Autodesk Inventor part; units mm, degrees
ref_plane "Work Plane1" through (0, 0, -15) normal (0, 0, 1) x (1, 0, 0)
ref_plane "YZ Plane" through (0, 0, 0) normal (1, 0, 0) x (0, 1, 0)
ref_plane "XZ Plane" through (0, 0, 0) normal (0, 1, 0) x (-1, 0, 0)
sketch "Sketch1" plane through (0, 0, 0) normal (0, 0, 1) x (1, 0, 0)
  line L0 (0, 0) -> (25, 0)
  line L1 (25, 0) -> (25, 40)
  line L2 (25, 40) -> (0, 40)
  line L3 (0, 40) -> (0, 0)
  dimension "d1" = 25
  dimension "d2" = 40
  dimension "d3" = 25
extrude "Extrusion1" add sketch "Sketch1" against normal blind 30
sketch "Sketch2" plane through (25, 0, 0) normal (1, 0, 0) x (0, 0, -1)
  line L0 (0, 0) -> (30, 0)
  circle A0 centre (15, 6.56) radius 2.46
extrude "Extrusion2" cut sketch "Sketch2" against normal blind 30
sketch "Sketch3" plane through (0, 0, 0) normal (-1, 0, 0) x (0, 0, 1)
  line L0 (0, 0) -> (-30, 0)
  line L1 (-25.05, 0) -> (-4.95, 0)
  line L2 (-4.95, 0) -> (-4.95, 33.12)
  line L3 (-4.95, 33.12) -> (-25.05, 33.12)
  line L4 (-25.05, 33.12) -> (-25.05, 0)
  dimension "d11" = 20.1
extrude "Extrusion3" cut sketch "Sketch3" against normal blind 20
sketch "Sketch4" plane through (0, 0, 0) normal (0, -1, 0) x (1, 0, 0)
  line L0 (20, -4.95) -> (20, -25.05)
  line L1 (20, -15) -> (25, -15)
  line L2 (25, 0) -> (25, -30)
  line L3 (20, -8.025) -> (25, -8.025)
  line L4 (25, -8.025) -> (25, -21.975)
  line L5 (25, -21.975) -> (20, -21.975)
  line L6 (20, -21.975) -> (20, -8.025)
  line L7 (20, -8.025) -> (25, -21.975) construction
  line L8 (25, -8.025) -> (20, -21.975) construction
  line L9 (25, -12.54) -> (25, -17.46)
  point P0 (0, 0)
  point P1 (22.5, -15)
  dimension "d14" = 13.95
extrude "Extrusion4" add sketch "Sketch4" along normal blind 15
sketch "Sketch5" plane through (20, 0, 0) normal (-1, 0, 0) x (0, 0, 1)
  circle A0 centre (-15, 6.56) radius 2.46
  circle A1 centre (-15, 6.56) radius 4.7025
  circle A2 centre (-15, 6.56) radius 2.46
  circle A3 centre (-15, 6.56) radius 2.46
  point P0 (0, 0)
  dimension "d17" = 9.405
extrude "Extrusion5" cut sketch "Sketch5" against normal blind 2.1
sketch "Sketch6" plane through (25, 0, 0) normal (1, 0, 0) x (0, 0, -1)
  circle A0 centre (15, 6.56) radius 4.7025
  line L0 (15, 6.56) -> (15, 23.56)
  circle A1 centre (15, 23.56) radius 2.46
  point P0 (0, 0)
  dimension "d20" = 17
  dimension "d21" = 4.92
extrude "Extrusion6" cut sketch "Sketch6" against normal blind 10 contours A1
sketch "Sketch7" plane through (20, 0, 0) normal (-1, 0, 0) x (0, 0, 1)
  circle A0 centre (-15, 23.56) radius 2.46
  circle A1 centre (-15, 23.56) radius 4.7025
  point P0 (0, 0)
  dimension "d24" = 9.405
extrude "Extrusion7" cut sketch "Sketch7" against normal blind 2.1
sketch "Sketch9" plane through (25, 0, 0) normal (1, 0, 0) x (0, 0, -1)
  circle A0 centre (15, 6.56) radius 2.46
  circle A1 centre (15, 6.56) radius 2.46
  circle A2 centre (15, 23.56) radius 2.46
  circle A3 centre (15, 23.56) radius 2.46
  line L0 (30, 40) -> (30, 0)
  line L1 (30, 0) -> (30, 40)
  line L2 (30, 40) -> (0, 40)
  line L3 (0, 40) -> (0, 0)
  line L4 (0, 0) -> (8.025, 0)
  line L5 (21.975, 0) -> (21.975, -15)
  line L6 (21.975, -15) -> (8.025, -15)
  line L7 (8.025, -15) -> (8.025, 0)
  line L8 (0, 0) -> (8.025, 0)
  line L9 (21.975, 0) -> (30, 0)
extrude "Extrusion8" add sketch "Sketch9" along normal blind 5
sketch "Sketch10" plane through (0, 40, 0) normal (0, 1, 0) x (1, 0, 0)
  line L0 (0, 30) -> (30, 30)
  line L1 (30, 0) -> (0, 0)
  line L2 (0, 30) -> (30, 30)
  line L3 (30, 30) -> (30, 0)
  line L4 (30, 0) -> (0, 0)
  line L5 (0, 0) -> (0, 30)
extrude "Extrusion9" add sketch "Sketch10" along normal blind 30
sketch "Sketch12" plane through (30, 0, 0) normal (1, 0, 0) x (0, 0, -1)
  circle A0 centre (15, 6.56) radius 2.46
  line L0 (15, 6.56) -> (15, 15.06)
  circle A1 centre (15, 15.06) radius 2.525
  point P0 (0, 0)
  dimension "d31" = 8.5
  dimension "d33" = 5.05
extrude "Extrusion10" cut sketch "Sketch12" against normal blind 30 contours A1
sketch "Sketch14" plane through (0, 0, 0) normal (0, 0, 1) x (1, 0, 0)
  line L0 (30, 70) -> (0, 70)
  line L1 (0, 70) -> (0, 85)
  line L2 (30, 0) -> (30, 70)
  line L3 (30, 122.5) -> (30, 70)
  line L4 (30, 105) -> (30, 100)
  line L5 (-12, 153) -> (15, 153)
  line L6 (-7, 150.5) -> (-12, 153)
  line L7 (-7, 102.5) -> (-12, 100)
  line L8 (-7, 102.5) -> (-2, 126.5)
  line L9 (-2, 126.5) -> (-7, 150.5)
  line L10 (30, 126.5) -> (15, 153)
  line L11 (30, 122.5) -> (30, 126.5)
  line L12 (0, 85) -> (0, 100)
  line L13 (0, 100) -> (-12, 100)
  point P0 (0, 0)
  dimension "d90" = 12
extrude "Extrusion12" add sketch "Sketch14" against normal blind 30
sketch "Sketch15" plane through (0, 0, -25.05) normal (-1, 0, 0) x (0, 0, 1)
  line L0 (0, 33.12) -> (20.1, 33.12)
  line L1 (20.1, 33.12) -> (20.1, 0)
  line L2 (0, 33.12) -> (20.1, 33.12)
  line L3 (20.1, 33.12) -> (20.1, 31.1)
  line L4 (20.1, 31.1) -> (0, 31.1)
  line L5 (0, 31.1) -> (0, 33.12)
  point P0 (25.05, 0)
  dimension "d57" = 2.02
extrude "Extrusion13" add sketch "Sketch15" against normal blind 20
sketch "Sketch25" plane through (0, 0, 0) normal (0, 0, 1) x (1, 0, 0)
  line L0 (0, 100) -> (-12, 100)
  line L1 (0, 100) -> (-12, 100)
  line L2 (-12, 100) -> (-7, 102.5)
  line L3 (-12, 100) -> (-7, 102.5)
  line L4 (-7, 102.5) -> (-2, 126.5)
  line L5 (-7, 102.5) -> (-2, 126.5)
  line L6 (-2, 126.5) -> (-7, 150.5)
  line L7 (-2, 126.5) -> (-7, 150.5)
  line L8 (-7, 150.5) -> (-12, 153)
  line L9 (-7, 150.5) -> (-12, 153)
  line L10 (-12, 153) -> (15, 153)
  line L11 (-12, 153) -> (15, 153)
  line L12 (15, 153) -> (30, 126.5)
  line L13 (15, 153) -> (30, 126.5)
  line L14 (30, 126.5) -> (30, 86.5)
  line L15 (30, 0) -> (30, 126.5)
  line L16 (30, 86.5) -> (0, 86.5)
  line L17 (0, 100) -> (0, 0)
  line L18 (0, 86.5) -> (0, 100)
  dimension "d91" = 40
  dimension "d92" = 30
extrude "Extrusion14" add sketch "Sketch25" along normal blind 45
ref_plane "Work Plane1" through (0, 0, -15) normal (0, 0, 1) x (1, 0, 0)
mirror "Mirror1" about plane through (0, 0, -15) normal (0, 0, 1) of "Extrusion14"
properties part number "rec_b_48mm_x_120mm"
Work out the finished part from the listing and answer in its coordinate system (mm). A direction names the side the tool comes from. Round coordinates to 2 decimals unless told otherwise and drop trailing zeros. Loops run counter-clockwise (first coordinate to the right, second up) from the corner with the lowest first, then second, coordinate; pieces in that order, holes last. Notation, with made-up numbers: (9.5, 57) - (15.5, 57) arc R30 cw to (15.5, 81) - close; hole circle Ø11 at (-28, 35). An arc over 180 degrees is marked (long way). One line per item, written item: value.
Q1. Find section A-A on z = -15. State how many separate pieces and enclosed holes the cut face has, and give its area (3 significant figures).
Check values:
separate pieces: 4
enclosed holes: 0
area: 4,020 mm2
Q2. Find section B-B on y = 15.06. Give the vertices of the cut face in (x, z) (3 decimals).
Check values:
outline: (0, -30) - (30, -30) - (30, -17.525) - (20, -17.525) - (20, -25.05) - (0, -25.05) - close; (0, -4.95) - (20, -4.95) - (20, -12.475) - (30, -12.475) - (30, 0) - (0, 0) - close
Q3. The mould has two halves that part along Y. Classify faces 5 (the flat face through (10, 31.1, -15)), 6 (the flat face through (-4.465, 114.668, -14.16)), 7 (the flat face through (22.1, 4.5, -13)), 8 (the flat face through (13, 120, 45)): +Y half, -Y half, draft (parallel to the pull), parting line (faces both ways), or undercut.
Check values:
face 5: -Y half
face 6: undercut
face 7: undercut
face 8: draft
Q4. Each of these flat-tipped pins is pushed along its axis until it touches: pin 1 Ø1 at (y, z) = (30, 0) entering from -X; pin 2 Ø24 at (x, y) = (10.5, 41.5) entering from -Z; pin 3 Ø7.5 at (y, z) = (23.5, -17) entering from -X; pin 4 Ø4.5 at (y, z) = (6.56, -15) entering from +X. Where does it stop, or does it pass through?
Check values:
pin 1: x = 0
pin 2: z = -30
pin 3: x = 20
pin 4: through
Q5. Find section C-C on x = 24.5. Give the vertices of the cut face in (y, z) (3 decimals), and give its area (3 significant figures).
Check values:
outline: (-15, -21.975) - (0, -21.975) - (0, -30) - (86.5, -30) - (86.5, -75) - (136.217, -75) - (136.217, 45) - (86.5, 45) - (86.5, 0) - (0, 0) - (0, -8.025) - (-15, -8.025) - close; hole circle Ø4.92 at (6.56, -15); hole circle Ø5.05 at (15.06, -15); hole circle Ø4.92 at (23.56, -15)
area: 8,710 mm2
Q6. For faces 1 (the flat face through (10, 15, -4.95)), 2 (the flat face through (22.1, 21.5, -13)), 3 (the flat face through (-10, 152, -14)), 4 (the flat face through (15, 44, 0)), determine the directions among +Z, -Z, +X, -X, +Y, -Y from which every point of the face is accessible in a straight line to the end or side of a thin tool.
Check values:
face 1: -X, -Y
face 2: -X
face 3: +Z, -Z, -X
face 4: +Z, +X, -X, -Y
Q7. Straight lines are drawn through the part: probe 1 along Y at (x, z) = (25, -15) (3 decimals); probe 2 along Y at (x, z) = (26, -15) (3 decimals); probe 3 along Z at (x, y) = (21, 23). For each, find the intervals that lie inside material, in ascending order.
Check values:
probe 1: -15 to 4.1, 9.02 to 12.535, 17.585 to 21.1, 26.02 to 135.333
probe 2: -15 to 4.1, 9.02 to 12.535, 17.585 to 21.1, 26.02 to 133.567
probe 3: -30 to -19.67, -10.33 to 0
Q8. Find section D-D on z = -33. Give the vertices of the cut face in (x, y).
Check values:
outline: (-12, 100) - (0, 100) - (0, 86.5) - (30, 86.5) - (30, 126.5) - (15, 153) - (-12, 153) - (-7, 150.5) - (-2, 126.5) - (-7, 102.5) - close
